Work out the finished part from the listing and answer in its coordinate system (mm). A direction names the side the tool comes from. Round coordinates to 2 decimals unless told otherwise and drop trailing zeros. Order: outer loops, then holes, each group sorted by start corner. A loop starts at its lowest first (then second) coordinate and runs counter-clockwise, first axis right, second up. Notation, with made-up numbers: (22.25, 39) -> (57.25, 39) arc R25 ccw to (57.25, 55) -> close; hole circle Ø10 at (-13, 57). An arc over 180 degrees is marked (long way). Use one line per item in the form item = value.
```python
from build123d import *

# Parameters (mm, degrees)
BOSS_EXTRUDE1_DEPTH = 2
SKETCH6_R           = 3.9
BOSS_EXTRUDE3_DEPTH = 3.5
CUT_EXTRUDE3_DEPTH  = 3.5
FILLET2_R           = 1
SKETCH8_R           = 0.75
CUT_EXTRUDE4_DEPTH  = 30.201883501
SKETCH9_R           = 1.5
CUT_EXTRUDE5_DEPTH  = 30.201883501


with BuildPart() as part:
    # Sketch1 → Boss-Extrude1 (new body)
    with BuildSketch(Plane(origin=(0, 0, 0), x_dir=(1, 0, 0), z_dir=(0, 1, 0))):
        with BuildLine():
            Line((-4, 4), (-1.479915293, 19.244644078))
            ThreePointArc((-1.479915293, 19.244644078), (0, 20.5), (1.479915293, 19.244644078))
            Line((1.479915293, 19.244644078), (4, 4))
            Line((4, 4), (19.244644078, 1.479915293))
            ThreePointArc((19.244644078, 1.479915293), (20.5, 0), (19.244644078, -1.479915293))
            Line((19.244644078, -1.479915293), (4, -4))
            Line((4, -4), (1.479915293, -19.244644078))
            ThreePointArc((1.479915293, -19.244644078), (0, -20.5), (-1.479915293, -19.244644078))
            Line((-1.479915293, -19.244644078), (-4, -4))
            Line((-4, -4), (-19.244644078, -1.479915293))
            ThreePointArc((-19.244644078, -1.479915293), (-20.5, 0), (-19.244644078, 1.479915293))
            Line((-19.244644078, 1.479915293), (-4, 4))
        make_face()
    extrude(amount=BOSS_EXTRUDE1_DEPTH)

    # Sketch6 → Boss-Extrude3 (add)
    with BuildSketch(Plane(origin=(0, 2, 0), x_dir=(1, 0, 0), z_dir=(0, 1, 0))):
        with Locations(Location((0, 0, 0), (0, 0, 270))):
            Circle(SKETCH6_R)
    extrude(amount=BOSS_EXTRUDE3_DEPTH)

    # Sketch7 → Cut-Extrude3 (cut)
    with BuildSketch(Plane(origin=(0, 5.5, 0), x_dir=(1, 0, 0), z_dir=(0, 1, 0))):
        with BuildLine():
            Line((0, 2.55), (-0.331043275, 2.881043275))
            ThreePointArc((-0.331043275, 2.881043275), (-0.363466377, 2.877132634), (-0.395843385, 2.872857117))
            Line((-0.395843385, 2.872857117), (-0.634159212, 2.469887061))
            Line((-0.634159212, 2.469887061), (-1.037129268, 2.708202888))
            ThreePointArc((-1.037129268, 2.708202888), (-1.067561203, 2.696351809), (-1.09785775, 2.684158781))
            Line((-1.09785775, 2.684158781), (-1.228471869, 2.234582034))
            Line((-1.228471869, 2.234582034), (-1.678048616, 2.365196153))
            ThreePointArc((-1.678048616, 2.365196153), (-1.704577232, 2.346149284), (-1.730889674, 2.326804877))
            Line((-1.730889674, 2.326804877), (-1.74559512, 1.85887))
            Line((-1.74559512, 1.85887), (-2.213529997, 1.873575446))
            ThreePointArc((-2.213529997, 1.873575446), (-2.234488404, 1.84852957), (-2.255163435, 1.823249265))
            Line((-2.255163435, 1.823249265), (-2.15303621, 1.366358327))
            Line((-2.15303621, 1.366358327), (-2.609927148, 1.264231103))
            ThreePointArc((-2.609927148, 1.264231103), (-2.623998452, 1.234759946), (-2.637736982, 1.205132197))
            Line((-2.637736982, 1.205132197), (-2.425194117, 0.787993336))
            Line((-2.425194117, 0.787993336), (-2.842332978, 0.57545047))
            ThreePointArc((-2.842332978, 0.57545047), (-2.848633027, 0.543405812), (-2.854571815, 0.51129224))
            Line((-2.854571815, 0.51129224), (-2.544968157, 0.160115825))
            Line((-2.544968157, 0.160115825), (-2.896144573, -0.149487832))
            ThreePointArc((-2.896144573, -0.149487832), (-2.894277512, -0.182092507), (-2.892043401, -0.214674088))
            Line((-2.892043401, -0.214674088), (-2.504832489, -0.477822352))
            Line((-2.504832489, -0.477822352), (-2.767980753, -0.865033264))
            ThreePointArc((-2.767980753, -0.865033264), (-2.758063897, -0.896149284), (-2.747797265, -0.927151654))
            Line((-2.747797265, -0.927151654), (-2.307308984, -1.085737193))
            Line((-2.307308984, -1.085737193), (-2.465894523, -1.526225475))
            ThreePointArc((-2.465894523, -1.526225475), (-2.448550984, -1.553897705), (-2.430896921, -1.581372872))
            Line((-2.430896921, -1.581372872), (-1.964808769, -1.625431174))
            Line((-1.964808769, -1.625431174), (-2.008867071, -2.091519326))
            ThreePointArc((-2.008867071, -2.091519326), (-1.985186607, -2.11400902), (-1.961254383, -2.136230616))
            Line((-1.961254383, -2.136230616), (-1.498852393, -2.062993336))
            Line((-1.498852393, -2.062993336), (-1.425615113, -2.525395325))
            ThreePointArc((-1.425615113, -2.525395325), (-1.397085655, -2.541289372), (-1.368379019, -2.556861134))
            Line((-1.368379019, -2.556861134), (-0.938717609, -2.370930039))
            Line((-0.938717609, -2.370930039), (-0.752786514, -2.800591449))
            ThreePointArc((-0.752786514, -2.800591449), (-0.721200673, -2.808891167), (-0.689523369, -2.816834664))
            Line((-0.689523369, -2.816834664), (-0.319599746, -2.529892488))
            Line((-0.319599746, -2.529892488), (-0.03265757, -2.899816112))
            ThreePointArc((-0.03265757, -2.899816112), (0, -2.9), (0.03265757, -2.899816112))
            Line((0.03265757, -2.899816112), (0.319599746, -2.529892488))
            Line((0.319599746, -2.529892488), (0.689523369, -2.816834664))
            ThreePointArc((0.689523369, -2.816834664), (0.721200673, -2.808891167), (0.752786514, -2.800591449))
            Line((0.752786514, -2.800591449), (0.938717609, -2.370930039))
            Line((0.938717609, -2.370930039), (1.368379019, -2.556861134))
            ThreePointArc((1.368379019, -2.556861134), (1.397085655, -2.541289372), (1.425615113, -2.525395325))
            Line((1.425615113, -2.525395325), (1.498852393, -2.062993336))
            Line((1.498852393, -2.062993336), (1.961254383, -2.136230616))
            ThreePointArc((1.961254383, -2.136230616), (1.985186607, -2.11400902), (2.008867071, -2.091519326))
            Line((2.008867071, -2.091519326), (1.964808769, -1.625431174))
            Line((1.964808769, -1.625431174), (2.430896921, -1.581372872))
            ThreePointArc((2.430896921, -1.581372872), (2.448550984, -1.553897705), (2.465894523, -1.526225475))
            Line((2.465894523, -1.526225475), (2.307308984, -1.085737193))
            Line((2.307308984, -1.085737193), (2.747797265, -0.927151654))
            ThreePointArc((2.747797265, -0.927151654), (2.758063897, -0.896149284), (2.767980753, -0.865033264))
            Line((2.767980753, -0.865033264), (2.504832489, -0.477822352))
            Line((2.504832489, -0.477822352), (2.892043401, -0.214674088))
            ThreePointArc((2.892043401, -0.214674088), (2.894277512, -0.182092507), (2.896144573, -0.149487832))
            Line((2.896144573, -0.149487832), (2.544968157, 0.160115825))
            Line((2.544968157, 0.160115825), (2.854571815, 0.51129224))
            ThreePointArc((2.854571815, 0.51129224), (2.848633027, 0.543405812), (2.842332978, 0.57545047))
            Line((2.842332978, 0.57545047), (2.425194117, 0.787993336))
            Line((2.425194117, 0.787993336), (2.637736982, 1.205132197))
            ThreePointArc((2.637736982, 1.205132197), (2.623998452, 1.234759946), (2.609927148, 1.264231103))
            Line((2.609927148, 1.264231103), (2.15303621, 1.366358327))
            Line((2.15303621, 1.366358327), (2.255163435, 1.823249265))
            ThreePointArc((2.255163435, 1.823249265), (2.234488404, 1.84852957), (2.213529997, 1.873575446))
            Line((2.213529997, 1.873575446), (1.74559512, 1.85887))
            Line((1.74559512, 1.85887), (1.730889674, 2.326804877))
            ThreePointArc((1.730889674, 2.326804877), (1.704577232, 2.346149284), (1.678048616, 2.365196153))
            Line((1.678048616, 2.365196153), (1.228471869, 2.234582034))
            Line((1.228471869, 2.234582034), (1.09785775, 2.684158781))
            ThreePointArc((1.09785775, 2.684158781), (1.067561203, 2.696351809), (1.037129268, 2.708202888))
            Line((1.037129268, 2.708202888), (0.634159212, 2.469887061))
            Line((0.634159212, 2.469887061), (0.395843385, 2.872857117))
            ThreePointArc((0.395843385, 2.872857117), (0.363466377, 2.877132634), (0.331043275, 2.881043275))
            Line((0.331043275, 2.881043275), (0, 2.55))
        make_face()
    extrude(amount=-CUT_EXTRUDE3_DEPTH, mode=Mode.SUBTRACT)

    # Fillet2
    fillet2_edges = [part.edges().sort_by_distance(p)[0] for p in [
        (-4, 1, -4),
        (4, 1, -4),
        (4, 1, 4),
        (-4, 1, 4),
    ]]
    fillet(fillet2_edges, radius=FILLET2_R)

    # Sketch8 → Cut-Extrude4 (cut, through all)
    with BuildSketch(Plane(origin=(0, 2, 0), x_dir=(1, 0, 0), z_dir=(0, 1, 0))):
        with Locations(Location((0, 16.5, 0), (0, 0, 270))):
            Circle(SKETCH8_R)
        with Locations(Location((0, 13.5, 0), (0, 0, 270))):
            Circle(SKETCH8_R)
        with Locations(Location((0, 10.5, 0), (0, 0, 270))):
            Circle(SKETCH8_R)
        with Locations(Location((0, 7, 0), (0, 0, 270))):
            Circle(SKETCH8_R)
        with Locations(Location((16.5, 0, 0), (0, 0, 270))):
            Circle(SKETCH8_R)
        with Locations(Location((13.5, 0, 0), (0, 0, 270))):
            Circle(SKETCH8_R)
        with Locations(Location((10.5, 0, 0), (0, 0, 270))):
            Circle(SKETCH8_R)
        with Locations(Location((7, 0, 0), (0, 0, 270))):
            Circle(SKETCH8_R)
        with Locations(Location((0, -16.5, 0), (0, 0, 270))):
            Circle(SKETCH8_R)
        with Locations(Location((0, -13.5, 0), (0, 0, 270))):
            Circle(SKETCH8_R)
        with Locations(Location((0, -10.5, 0), (0, 0, 270))):
            Circle(SKETCH8_R)
        with Locations(Location((0, -7, 0), (0, 0, 270))):
            Circle(SKETCH8_R)
        with Locations(Location((-16.5, 0, 0), (0, 0, 270))):
            Circle(SKETCH8_R)
        with Locations(Location((-13.5, 0, 0), (0, 0, 270))):
            Circle(SKETCH8_R)
        with Locations(Location((-10.5, 0, 0), (0, 0, 270))):
            Circle(SKETCH8_R)
        with Locations(Location((-7, 0, 0), (0, 0, 270))):
            Circle(SKETCH8_R)
    extrude(amount=-CUT_EXTRUDE4_DEPTH, mode=Mode.SUBTRACT)

    # Sketch9 → Cut-Extrude5 (cut, through all)
    with BuildSketch(Plane(origin=(0, 2, 0), x_dir=(1, 0, 0), z_dir=(0, 1, 0))):
        with Locations(Location((0, 0, 0), (0, 0, 270))):
            Circle(SKETCH9_R)
    extrude(amount=-CUT_EXTRUDE5_DEPTH, mode=Mode.SUBTRACT)


solid = part.part
```
Item 1: Determine the mould class of faces 1 (the flat face through (-3, 5.5, -1)), 2 (the cylindrical face through (0.03, 1.01, -14.25)), 3 (the flat face through (2.665, 0.986, -12.077)) for opening direction Z: released by +Z, released by -Z, zero draft, split by the parting line, or undercut.
Findings:
face_1 = zero draft
face_2 = undercut
face_3 = released by -Z
Item 2: Flat-ended cylindrical pins translate along their axes: P1, Ø2, axis at x = 0, z = -13.5, coming from the -Y side; P2, Ø3, axis at x = 9, y = 1.5, coming from the +Z side; P3, Ø3, axis at x = 12, z = 6, coming from the +Y side; P4, Ø1.5, axis at x = -5, y = 2, coming from the -Z side (3 decimals). Find the tip coordinate at first contact, or state that the pin passes through.
Findings:
P1 = 0
P2 = 3.42
P3 = through
P4 = -4.085
Item 3: For faces 4 (the cylindrical face through (7.225, 1.014, 0.715)), 5 (the cylindrical face through (-2.373, 3.726, -3.095)), determine the directions among +Z, -Z, +X, -X, +Y, -Y from which every point of the face is accessible in a straight line to the end or side of a thin tool.
Findings:
face_4 = +Y, -Y
face_5 = +Y
Item 4: Consider line 1 along X through (y, z) = (0.75, 13.5); line 2 along X through (y, z) = (0.2, 17); line 3 along Y through (x, z) = (7, -1). Determine where each line is inside the solid, lowest interval first.
Findings:
line_1 = -2.43 to -0.75, 0.75 to 2.43
line_2 = -1.85 to -0.56, 0.56 to 1.85
line_3 = 0 to 2
Item 5: The part is cut by section A-A, the plane z = -16.5. Give the vertices of the cut face in (x, y), and give its area (3 significant figures).
Findings:
outline = (-1.93, 0) -> (-0.75, 0) -> (-0.75, 2) -> (-1.93, 2) -> close; (0.75, 0) -> (1.93, 0) -> (1.93, 2) -> (0.75, 2) -> close
area = 4.73 mm^2
Item 6: The part is cut by section B-B, the plane x = 13.5. Give the vertices of the cut face in (y, z), and give its area (3 significant figures).
Findings:
outline = (0, -2.43) -> (2, -2.43) -> (2, -0.75) -> (0, -0.75) -> close; (0, 0.75) -> (2, 0.75) -> (2, 2.43) -> (0, 2.43) -> close
area = 6.72 mm^2
Item 7: The part is cut by section C-C, the plane y = 0.8. Give the number of separate pieces and of enclosed holes in the cut face, and give its area (3 significant figures).
Findings:
separate_pieces = 1
enclosed_holes = 17
area = 374 mm^2
